Work out the finished part from the listing and answer in its coordinate system (mm). A direction names the side the tool comes from. Coordinates: 2 decimals unless noted, no trailing zeros. Order: outer loops, then holes, each group sorted by start corner. A loop starts at its lowest first (then second) coordinate and runs counter-clockwise, first axis right, second up.
```python
from build123d import *


with BuildPart() as f1:
    # F0 (on Front) → F1 (revolve)
    with BuildSketch(Plane.XZ):
        with BuildLine():
            Line((0, 8.75), (0, 0))
            Line((0, 0), (108.719505762, 0))
            Line((108.719505762, 0), (108.719505762, 17.5))
            Line((108.719505762, 17.5), (68.719505762, 17.5))
            Line((68.719505762, 17.5), (68.719505762, 30))
            Line((68.719505762, 30), (55.7926830174, 30))
            ThreePointArc((55.7926830174, 30), (54.3784694551, 29.4142135624), (53.7926830174, 28))
            Line((53.7926830174, 28), (53.7926830174, 23.75))
            add(Edge.make_bspline(
                [(0, 8.75), (5.0406153604, 9.0258980354), (16.3424850669, 9.5343195461), (38.0075656916, 5.0292358393), (49.6364947054, 17.2036020787), (53.7926830174, 23.75)],
                knots=[0, 0, 0, 0, 0.3026453885, 0.6427893554, 1, 1, 1, 1], degree=3))
        make_face()
    revolve(axis=Axis((54.359752881, 0, 0), (-1, 0, 0)))

    # F2: F1 across face


with BuildPart() as f1_1:
    add(f1.part)
    add(f1.part.mirror(Plane(origin=(0, 0, 0), x_dir=(0, -1, 0), z_dir=(-1, 0, 0))))


solid = f1_1.part
```
1. Flat-ended cylindrical pins translate along their axes: pin 1 (4 mm diameter, centred on x = -42, z = 10, fed in from -Y); pin 2 (12 mm diameter, centred on x = -51, z = 4.5, fed in from -Y); pin 3 (5 mm diameter, centred on x = -36, z = -3.5, fed in from -Y). Find the tip coordinate at first contact, or state that the pin passes through.
2. The mould has two halves that part along X. Classify faces 4 (the cylindrical face through (-62.17, 1.32, -29.97)), 5 (the flat face through (53.793, -21, -13)), 6 (the flat face through (-53.793, -21, -13)), 7 (the flat face through (108.72, 0, 0)): released by +X, released by -X, zero draft, split by the parting line, or undercut.
3. Consider probe 1 along X at (y, z) = (22, 14.5); probe 2 along X at (y, z) = (-18, 2); probe 3 along Z at (x, y) = (-41.5, 4). Determine where each line is inside the solid, lowest interval first.
4. The part is cut by section B-B (x = -71.5). Determine the outline of the cut face in (y, z).
5. The part is cut by section A-A (y = 9). Count the separate pieces of the cut face and the enclosed holes in it, plus the area to 3 significant figures.
6. For faces 1 (the flat face through (68.72, -13, -13)), 2 (the flat face through (-108.72, 0, 0)), 3 (the cylindrical face through (-88.44, -10.648, -13.887)), determine the directions among +Z, -Z, +X, -X, +Y, -Y from which every point of the face is accessible in a straight line to the end or side of a thin tool.
Worked out:
1. pin 1: stops at y = -8.7
1. pin 2: stops at y = -29.99
1. pin 3: stops at y = -8.97
2. face 4: zero draft
2. face 5: undercut
2. face 6: undercut
2. face 7: released by +X
3. probe 1: x = -68.72 to -53.79, 53.79 to 68.72
3. probe 2: x = -68.72 to -49.65, 49.65 to 68.72
3. probe 3: z = -10.18 to 10.18
4. outline: circle Ø35 at (0, 0)
5. separate pieces: 4
5. enclosed holes: 0
5. area: 4,850 mm2
6. face 1: +X
6. face 2: +Z, -Z, -X, +Y, -Y
6. face 3: -X
